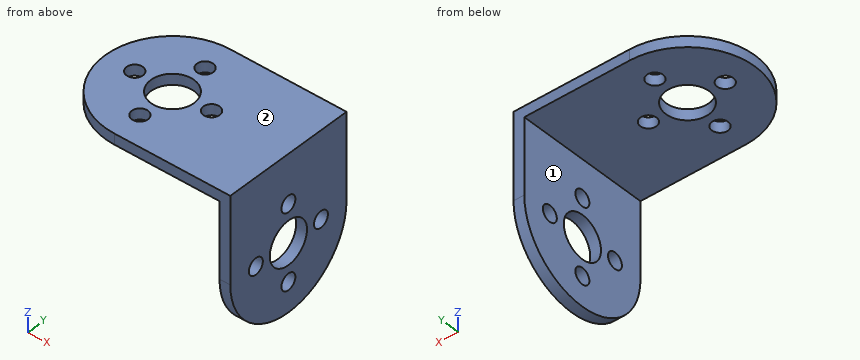
Autodesk Fusion 360 part; units mm, degrees
sketch "Boceto1" plane through (0, 0, 0) normal (0, 0, 1) x (1, 0, 0)
  line L0 (0, 12.5) -> (0, -12.5)
  arc A0 (0, 12.5) -> (0, -12.5) centre (0, 0) ccw
  line L1 (0, 12.5) -> (19.5, 12.5)
  line L2 (0, -12.5) -> (19.5, -12.5)
  line L3 (19.5, -12.5) -> (19.5, 12.5)
  circle A1 centre (0, 0) radius 4
  circle A2 centre (0, 0) radius 7 construction
  circle A3 centre (0, 7) radius 1.5
  circle A4 centre (-7, 0) radius 1.5
  circle A5 centre (0, -7) radius 1.5
  circle A6 centre (6.9935, 0.3006) radius 1.5
  dimension "d1" = 25
  dimension "d2" = 19.5
  dimension "d3" = 19.5
  dimension "d4" = 8
  dimension "d5" = 14
  dimension "d6" = 3
  dimension "d7" = 3
  dimension "d8" = 3
  dimension "d9" = 3
extrude "Extruir1" add sketch "Boceto1" along normal blind 2 contours L0 L1 L2 L3 A1 A3 A5 | L0 A0 A1 A3 A5
sketch "Boceto2" plane through (19.5, 0, 0) normal (1, 0, 0) x (0, 1, 0)
  line L0 (-12.5, 0) -> (12.5, 0)
  line L1 (12.5, 0) -> (12.5, 2)
  line L2 (12.5, 2) -> (-12.5, 2)
  line L3 (-12.5, 2) -> (-12.5, 0)
  line L4 (12.5, 0) -> (12.5, -14)
  line L5 (-12.5, 0) -> (-12.5, -14)
  circle A0 centre (0, -14) radius 4
  circle A1 centre (0, -14) radius 7 construction
  circle A2 centre (0, -7) radius 1.5
  circle A3 centre (-7, -14) radius 1.5
  circle A4 centre (0, -21) radius 1.5
  circle A5 centre (7, -14) radius 1.5
  circle A6 centre (0, -14) radius 12.5
  line L6 (-12.5, 2) -> (12.5, 2)
  line L7 (12.5, 2) -> (12.5, 0)
  line L8 (12.5, 0) -> (-12.5, 0)
  line L9 (-12.5, 0) -> (-12.5, 2)
  dimension "d12" = 14
  dimension "d13" = 14
  dimension "d14" = 8
  dimension "d15" = 14
  dimension "d16" = 3
  dimension "d17" = 3
  dimension "d18" = 3
  dimension "d19" = 3
extrude "Extruir2" add sketch "Boceto2" along normal blind 2
equation "d1 = ( 12.5 * 2 ) * 1 mm"
Input: part model. Units: mm. Frame: model coordinates. Face numbers are marked on the shaded views. A direction names the side the tool comes from. Coordinates: 2 decimals unless noted, no trailing zeros. Loops run counter-clockwise (first coordinate to the right, second up) from the corner with the lowest first, then second, coordinate; pieces in that order, holes last. Notation, with made-up numbers: (76, -30.5) -> (99, -30.5) arc R38 cw to (99, 8.5) -> close; hole circle Ø5 at (-22.5, 22). An arc over 180 degrees is marked (long way). One line per item, written item: value.
(1) Set-up query: the marked faces 1 and 2. Return all of +Z, -Z, +X, -X, +Y, -Y with unobstructed straight access to the full face (end or side cutting, diameter ignored); none if empty.
Answer below:
face 1: -Z, -X, +Y, -Y
face 2: +Z, +X, -X, +Y, -Y
(2) Pin query (flat end, axial travel): pin 1 Ø9 at (y, z) = (0, -14) entering from -X; pin 2 Ø1.8 at (y, z) = (0, -21) entering from -X; pin 3 Ø10 at (x, y) = (-5, 3.5) entering from -Z. Return the tip coordinate at first contact, or that it passes through.
Answer below:
pin 1: stops at x = 19.5
pin 2: passes through
pin 3: stops at z = 0
(3) Cut plane D-D (x = 1). Output: boundary loops of the cut face in (y, z).
Answer below:
outline: (-12.5, 0) -> (-8.12, 0) -> (-8.12, 2) -> (-12.5, 2) -> close; (-5.88, 0) -> (-3.87, 0) -> (-3.87, 2) -> (-5.88, 2) -> close; (3.87, 0) -> (5.88, 0) -> (5.88, 2) -> (3.87, 2) -> close; (8.12, 0) -> (12.5, 0) -> (12.5, 2) -> (8.12, 2) -> close
(4) Cut plane A-A (y = 7.75). Output: boundary loops of the cut face in (x, z).
Answer below:
outline: (-9.81, 0) -> (-1.3, 0) -> (-1.3, 2) -> (-9.81, 2) -> close; (1.3, 0) -> (19.5, 0) -> (19.5, -12.7) -> (21.5, -12.7) -> (21.5, 2) -> (1.3, 2) -> close; (19.5, -23.81) -> (21.5, -23.81) -> (21.5, -15.3) -> (19.5, -15.3) -> close
(5) Cut plane C-C (z = -17.5). Output: boundary loops of the cut face in (x, y).
Answer below:
outline: (19.5, -12) -> (21.5, -12) -> (21.5, -1.94) -> (19.5, -1.94) -> close; (19.5, 1.94) -> (21.5, 1.94) -> (21.5, 12) -> (19.5, 12) -> close
(6) Cut plane B-B (x = -7). Output: boundary loops of the cut face in (y, z).
Answer below:
outline: (-10.36, 0) -> (-1.5, 0) -> (-1.5, 2) -> (-10.36, 2) -> close; (1.5, 0) -> (10.36, 0) -> (10.36, 2) -> (1.5, 2) -> close
(7) Ray query, line 1 along Y through (x, z) = (0, 1.2); line 2 along Z through (x, y) = (20.4, 0); line 3 along Z through (x, y) = (11, 7.5). Return the intervals inside material, ascending.
Answer below:
line 1: y = -12.5 to -8.5, -5.5 to -4, 4 to 5.5, 8.5 to 12.5
line 2: z = -26.5 to -22.5, -19.5 to -18, -10 to -8.5, -5.5 to 2
line 3: z = 0 to 2
